Check sheet for the modelled part. Datum: model origin and axes. Units: mm. A direction names the side the tool comes from. Round coordinates to 2 decimals unless told otherwise and drop trailing zeros. Loops run counter-clockwise (first coordinate to the right, second up) from the corner with the lowest first, then second, coordinate; pieces in that order, holes last. Notation, with made-up numbers: (78.25, 50.5) - (137.25, 50.5) arc R21 cw to (137.25, 58.5) - close; hole circle Ø2 at (-21.5, 44.5). An arc over 180 degrees is marked (long way). Answer in a Markdown table with one row per item. Add a question column.
(1) Gauge pin test, flat ends, axial feed: pin 1 (15 mm diameter, centred on x = 13.5, z = -18.5, fed in from -Y); pin 2 (2 mm diameter, centred on y = 7.5, z = -6, fed in from -X); pin 3 (2 mm diameter, centred on y = 10.5, z = -9, fed in from -X); pin 4 (5 mm diameter, centred on y = 7, z = -15.5, fed in from +X). Record the tip position at first contact, or that the pin passes through.
(2) Mould release check, pull along X, two halves, no side actions. Record for faces 6 (the flat face through (13, 15.1, -14)), 7 (the flat face through (22.7, 5.8, -13.8)), 8 (the cylindrical face through (0.285, 14.101, -13.93)), 9 (the flat face through (3, 12, -14)): +X half, -X half, draft (parallel to the pull), parting line (faces both ways), or undercut.
(3) Thickness scan on line 1 along X through (y, z) = (6.75, -2.5); line 2 along X through (y, z) = (11.5, -22.75); line 3 along Y through (x, z) = (7.75, -22.25). Record the ranges inside material, lowest first.
(4) Cross-section at C-C on x = 20.75. Enter the section's corners in (y, z), then the cut area to 3 significant figures.
(5) Cross-section at A-A on z = -18. Enter the section's corners in (x, y).
(6) Access from +Z, -Z, +X, -X, +Y, -Y to the whole of each face (thin tool, end or side, straight path). Record for faces 1 (the cylindrical face through (25, 9.1, -23.8)), 2 (the flat face through (13, 17, -28)), 3 (the flat face through (1.5, 4.2, -13.9)), 4 (the flat face through (26.7, 17, -14)), 5 (the flat face through (23, 6, -14)).
(7) Cross-section at D-D on y = 11.25. Count the separate pieces of the cut face and the enclosed holes in it, then the cut area to 3 significant figures.
(8) Cross-section at B-B on y = 9. Enter the section's corners in (x, z).
from build123d import *

# Parameters (mm, degrees)
SKETCH1_W           = 26.7
SKETCH1_H           = 28
BOSS_EXTRUDE1_DEPTH = 20
CUT_EXTRUDE1_DEPTH  = 27.5
CUT_EXTRUDE2_DEPTH  = 2
CUT_EXTRUDE3_DEPTH  = 2.4
SKETCH5_W           = 18.7
SKETCH5_H           = 28
CUT_EXTRUDE4_DEPTH  = 15.1
FILLET1_R           = 1


with BuildPart() as part:
    # Sketch1 → Boss-Extrude1 (new body)
    with BuildSketch(Plane(origin=(0, 0, 0), x_dir=(1, 0, 0), z_dir=(0, 1, 0))):
        with Locations((13.35, 14)):
            Rectangle(SKETCH1_W, SKETCH1_H)
    extrude(amount=BOSS_EXTRUDE1_DEPTH)

    # Sketch2 → Cut-Extrude1 (cut)
    with BuildSketch(Plane.ZY):
        with BuildLine():
            Line((-19, 12), (-9, 12))
            ThreePointArc((-9, 12), (-6, 9), (-9, 6))
            Line((-9, 6), (-19, 6))
            ThreePointArc((-19, 6), (-22, 9), (-19, 12))
        make_face()
    extrude(amount=-CUT_EXTRUDE1_DEPTH, mode=Mode.SUBTRACT)

    # Sketch3 → Cut-Extrude2 (cut)
    with BuildSketch(Plane.ZY):
        with BuildLine():
            Line((-19, 13.8), (-9, 13.8))
            ThreePointArc((-9, 13.8), (-4.2, 9), (-9, 4.2))
            Line((-9, 4.2), (-19, 4.2))
            ThreePointArc((-19, 4.2), (-23.8, 9), (-19, 13.8))
        make_face()
    extrude(amount=-CUT_EXTRUDE2_DEPTH, mode=Mode.SUBTRACT)

    # Sketch4 → Cut-Extrude3 (cut)
    with BuildSketch(Plane(origin=(26.7, 0, 0), x_dir=(0, 0, -1), z_dir=(1, 0, 0))):
        with BuildLine():
            Line((9, 13.8), (19, 13.8))
            ThreePointArc((19, 13.8), (23.8, 9), (19, 4.2))
            Line((19, 4.2), (9, 4.2))
            ThreePointArc((9, 4.2), (4.2, 9), (9, 13.8))
        make_face()
    extrude(amount=-CUT_EXTRUDE3_DEPTH, mode=Mode.SUBTRACT)

    # Sketch5 → Cut-Extrude4 (cut)
    with BuildSketch(Plane(origin=(0, 0, 0), x_dir=(1, 0, 0), z_dir=(0, 1, 0))):
        with Locations((13.35, 14)):
            Rectangle(SKETCH5_W, SKETCH5_H)
    extrude(amount=CUT_EXTRUDE4_DEPTH, mode=Mode.SUBTRACT)

    # Fillet1
    fillet1_edges = [part.edges().sort_by_distance(p)[0] for p in [
        (0, 9, -23.8),
        (0, 4.2, -14),
        (0, 9, -4.2),
        (0, 13.8, -14),
        (26.7, 9, -4.2),
        (26.7, 4.2, -14),
        (26.7, 9, -23.8),
        (26.7, 13.8, -14),
    ]]
    fillet(fillet1_edges, radius=FILLET1_R)


solid = part.part
Answers:
| question | item | result |
|---|---|---|
| 1 | pin 1 | stops at y = 15.1 |
| 1 | pin 2 | stops at x = 2 |
| 1 | pin 3 | passes through |
| 1 | pin 4 | stops at x = 24.3 |
| 2 | face 6 | undercut |
| 2 | face 7 | undercut |
| 2 | face 8 | -X half |
| 2 | face 9 | draft |
| 3 | line 1 | x = 0 to 4, 22.7 to 26.7 |
| 3 | line 2 | x = 2 to 4, 22.7 to 24.3 |
| 3 | line 3 | y = 15.1 to 20 |
| 4 | outline | (15.1, -28) - (20, -28) - (20, 0) - (15.1, 0) - close |
| 4 | area | 137 mm^2 |
| 5 | outline | (0, 0) - (4, 0) - (4, 6) - (2, 6) - (2, 4.2) - (1, 4.2) arc R1 ccw to (0, 3.2) - close; (0, 14.8) arc R1 ccw to (1, 13.8) - (2, 13.8) - (2, 12) - (4, 12) - (4, 15.1) - (22.7, 15.1) - (22.7, 12) - (24.3, 12) - (24.3, 13.8) - (25.7, 13.8) arc R1 ccw to (26.7, 14.8) - (26.7, 20) - (0, 20) - close; (22.7, 0) - (26.7, 0) - (26.7, 3.2) arc R1 ccw to (25.7, 4.2) - (24.3, 4.2) - (24.3, 6) - (22.7, 6) - close |
| 6 | face 1 | +X |
| 6 | face 2 | -Z, +X, -X, +Y, -Y |
| 6 | face 3 | -X |
| 6 | face 4 | +Z, -Z, +X, +Y, -Y |
| 6 | face 5 | +X, -X |
| 7 | separate pieces | 4 |
| 7 | enclosed holes | 0 |
| 7 | area | 91.4 mm^2 |
| 8 | outline | (0, -28) - (4, -28) - (4, -22) - (2, -22) - (2, -23.8) - (1, -23.8) arc R1 ccw to (0, -24.8) - close; (0, -3.2) arc R1 ccw to (1, -4.2) - (2, -4.2) - (2, -6) - (4, -6) - (4, 0) - (0, 0) - close; (22.7, -28) - (26.7, -28) - (26.7, -24.8) arc R1 ccw to (25.7, -23.8) - (24.3, -23.8) - (24.3, -22) - (22.7, -22) - close; (22.7, -6) - (24.3, -6) - (24.3, -4.2) - (25.7, -4.2) arc R1 ccw to (26.7, -3.2) - (26.7, 0) - (22.7, 0) - close |
